Input: part model. Units: mm. Frame: model coordinates. Face numbers are marked on the shaded views. Round coordinates to 2 decimals unless told otherwise and drop trailing zeros. Loops run counter-clockwise (first coordinate to the right, second up) from the corner with the lowest first, then second, coordinate; pieces in that order, holes last. Notation, with made-up numbers: (-33, -14.75) -> (-28, -14.75) arc R23 cw to (-28, 17.25) -> close; hole circle Ø1 at (-9, -12). An arc over 180 degrees is marked (long way). Answer as a JSON object with one key per item and string values.
```python
from build123d import *

# Parameters (mm, degrees)
F0_R     = 21.8313
F1_DEPTH = 1.5875
F2_R     = 19.3793862589
F3_DEPTH = 3
F4_R     = 19.4142729727
F5_DEPTH = 3
F5_TAPER = -10
F6_R     = 20
F7_DEPTH = 30.1498
F8_T     = 1
F10_D    = 12.7


# Not quite as in the source:
# - a length typed as a fraction of an inch, garbled in the dataset ("3 / 203.2 mm" for 3/8 in), is restored
# - a shell that OpenCascade refuses in one call is made with other operations: the cavity is built on its own and cut out


with BuildPart() as f1:
    # F0 (on Top) → F1 (new body)
    with BuildSketch(Plane.XY):
        Circle(F0_R)
    extrude(amount=F1_DEPTH)

    # F2 (on face) → F3 (join)
    with BuildSketch(Plane.XY.offset(1.5875)):
        Circle(F2_R)
    extrude(amount=F3_DEPTH)

    # F4 (on face) → F5 (join)
    with BuildSketch(Plane.XY.offset(4.5875)):
        Circle(F4_R)
    extrude(amount=F5_DEPTH, taper=F5_TAPER)

    # F6 (on face) → F7 (join)
    with BuildSketch(Plane.XY.offset(7.5875)):
        Circle(F6_R)
    extrude(amount=F7_DEPTH)

    # F8: shell of thickness 1, made by hand


with BuildPart() as f8_core1:
    # F8_t2: copy of F1
    add(f1.part)

    # the walls: a layer under each face that stays
    f8_faces = [f8_core1.faces().sort_by_distance(p)[0] for p in [
        (-20, 0, 22.6624),
        (17.5, -9.6296296296, 7.5875),
        (-19.6787634438, 0, 6.0875),
        (16.9874888511, -9.3476129128, 4.5875),
        (-19.3793862589, 0, 3.0875),
        (-14.5542, -14.5542, 1.5875),
        (-21.8313, 0, 0.79375),
        (0, 0, 0),
    ]]
    thicken(f8_faces, amount=-F8_T, mode=Mode.SUBTRACT)

    # F8_s3 → F8_t4 (revolve, cut)
    with BuildSketch(Plane.XZ):
        Polygon((19.9531019924, 7.5757635182), (19.9432539149, 8.5875), (19.1041542837, 8.5875), (18.9584461618, 7.7611481777), align=None)
    revolve(axis=Axis((0, 0, 7.5875), (0, 0, -1)), mode=Mode.SUBTRACT)

    # F8_s5 → F8_t6 (revolve, cut)
    with BuildSketch(Plane.XZ):
        Polygon((19.3893862589, 4.5775), (19.3793862589, 5.5875), (18.3793862589, 5.5875), (18.3793862589, 4.5875), align=None)
    revolve(axis=Axis((0, 0, 4.5875), (0, 0, 1)), mode=Mode.SUBTRACT)

    # F8_s7 → F8_t8 (revolve, cut)
    with BuildSketch(Plane.XZ):
        Polygon((19.3893862589, 1.5975), (18.3793862589, 1.5875), (18.3793862589, 0.5875), (19.3793862589, 0.5875), align=None)
    revolve(axis=Axis((0, 0, 1.5875), (0, 0, 1)), mode=Mode.SUBTRACT)


with BuildPart() as f1_1:
    add(f1.part)

    # what is left inside the walls is the cavity
    f8_cavity = [f8_core1.part.solids().sort_by_distance(p)[0] for p in [
        (-18.99, 0, 27.823804),
    ]]
    add(f8_cavity, mode=Mode.SUBTRACT)

    # F10 (through all)
    with Locations(Plane(origin=(0, 0, 0), x_dir=(1, 0, 0), z_dir=(0, 0, -1))):
        with Locations((0, 0)):
            Hole(F10_D / 2)


solid = f1_1.part
```
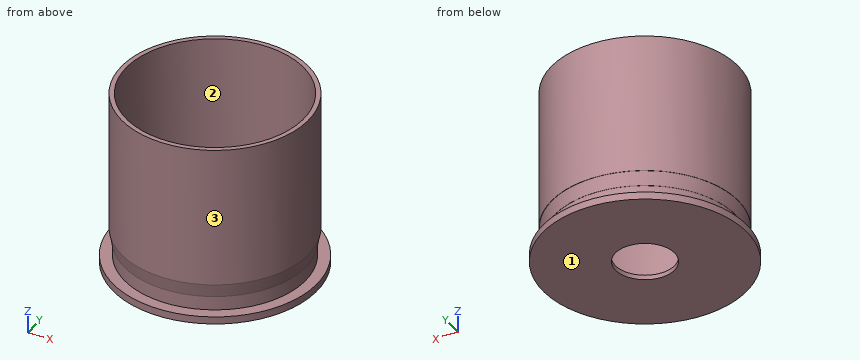
1) Section A-A, the plane z = 34. Output: boundary loops of the cut face in (x, y), plus the area to 3 significant figures.
Output:
{"outline": "circle Ø40 at (0, 0); hole circle Ø38 at (0, 0)", "area": "123 mm^2"}
2) Contact query for flat-ended pins moving along their axis: P1, Ø10, axis at x = -2.5, z = 6.5, coming from the +Y side; P2, Ø6, axis at x = -8, y = 2.5, coming from the -Z side; P3, Ø12, axis at x = 8.5, z = 8, coming from the +Y side; P4, Ø7.5, axis at x = 0, y = 0, coming from the +Z side. Output: stop coordinate, or through.
Output:
{"P1": "stops at y = 21.77", "P2": "stops at z = 0", "P3": "stops at y = 19.84", "P4": "passes through"}
3) Section B-B, the plane z = 7. Output: boundary loops of the cut face in (x, y), plus the area to 3 significant figures.
Output:
{"outline": "circle Ø39.68 at (0, 0); hole circle Ø37.65 at (0, 0)", "area": "123 mm^2"}
4) Draft query along Y for the marked faces 1, 2 and 3. Return one class per face: +Y half, -Y half, draft (parallel to the pull), parting line (faces both ways), or undercut.
Output:
{"face 1": "draft", "face 2": "undercut", "face 3": "parting line"}
5) Ray query, probe 1 along Y at (x, z) = (0, 26); probe 2 along Y at (x, z) = (0, 2.45); probe 3 along Z at (x, y) = (12.5, 5). Return the intervals inside material, ascending.
Output:
{"probe 1": "y = -20 to -19, 19 to 20", "probe 2": "y = -19.38 to -18.38, 18.38 to 19.38", "probe 3": "z = 0 to 1"}
